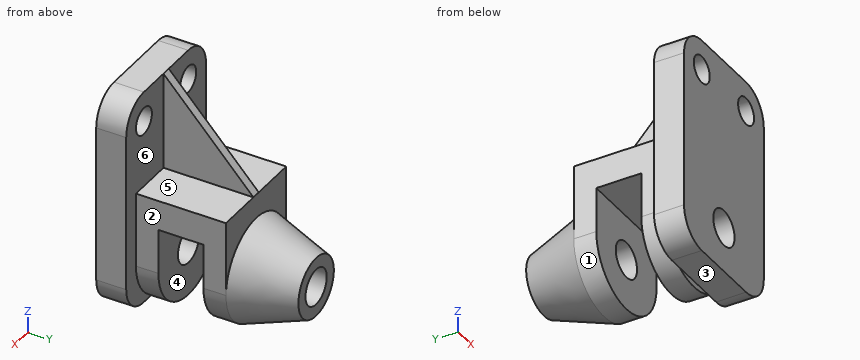
from build123d import *

# Parameters (mm, degrees)
SKETCH2_W           = 90
SKETCH2_H           = 145
SKETCH2_R           = 9
BOSS_EXTRUDE2_DEPTH = 20
FILLET1_R           = 20
FILLET2_R           = 20
BOSS_EXTRUDE3_DEPTH = 60
SKETCH4_W           = 83.251362913
SKETCH4_H           = 30
CUT_EXTRUDE1_DEPTH  = 136.98988933
SKETCH5_R           = 34
SKETCH6_R           = 20
SKETCH6_3_R         = 12
CUT_EXTRUDE2_DEPTH  = 150.255653211
RIB2_REACH          = 151.256
SKETCH9_WALL_W      = 388.970336646
SKETCH9_WALL_H      = 6


with BuildPart() as part:
    # Sketch2 → Boss-Extrude2 (new body)
    with BuildSketch(Plane(origin=(0, 0, 0), x_dir=(1, 0, 0), z_dir=(0, 1, 0))):
        Rectangle(SKETCH2_W, SKETCH2_H)
        with Locations(Location((-25, -52.5, 0), (0, 0, 270))):
            Circle(SKETCH2_R, mode=Mode.SUBTRACT)
        with Locations(Location((25, -52.5, 0), (0, 0, 270))):
            Circle(SKETCH2_R, mode=Mode.SUBTRACT)
    extrude(amount=BOSS_EXTRUDE2_DEPTH)

    # Fillet1
    fillet1_edges = [part.edges().sort_by_distance(p)[0] for p in [
        (45, 10, 72.5),
        (-45, 10, 72.5),
    ]]
    fillet(fillet1_edges, radius=FILLET1_R)

    # Fillet2
    fillet2_edges = [part.edges().sort_by_distance(p)[0] for p in [
        (-45, 10, -72.5),
        (45, 10, -72.5),
    ]]
    fillet(fillet2_edges, radius=FILLET2_R)

    # Sketch3 → Boss-Extrude3 (add)
    with BuildSketch(Plane(origin=(0, 20, 0), x_dir=(1, 0, 0), z_dir=(0, 1, 0))):
        with BuildLine():
            Line((-34, -7.5), (34, -7.5))
            Line((34, -7.5), (34, 42.5))
            ThreePointArc((34, 42.5), (0, 76.5), (-34, 42.5))
            Line((-34, 42.5), (-34, -7.5))
        make_face()
    extrude(amount=BOSS_EXTRUDE3_DEPTH)

    # Sketch4 → Cut-Extrude1 (cut, through all)
    with BuildSketch(Plane(origin=(34, 0, 0), x_dir=(0, 0, -1), z_dir=(1, 0, 0))):
        with Locations((54.125681457, 50)):
            Rectangle(SKETCH4_W, SKETCH4_H)
    extrude(amount=-CUT_EXTRUDE1_DEPTH, mode=Mode.SUBTRACT)

    # Sketch5 → Loft1 section 0
    with BuildSketch(Plane(origin=(0, 80, 0), x_dir=(1, 0, 0), z_dir=(0, 1, 0))):
        with Locations((0, 42.5)):
            Circle(SKETCH5_R)
    # Sketch6 → Loft1 section 1
    with BuildSketch(Plane(origin=(0, 120, 0), x_dir=(1, 0, 0), z_dir=(0, 1, 0))):
        with Locations((0, 42.5)):
            Circle(SKETCH6_R)
    loft()

    # Sketch6<3> → Cut-Extrude2 (cut, through all)
    with BuildSketch(Plane(origin=(0, 120, 0), x_dir=(1, 0, 0), z_dir=(0, 1, 0))):
        with Locations(Location((0, 42.5, 0), (0, 0, 270))):
            Circle(SKETCH6_3_R)
    extrude(amount=-CUT_EXTRUDE2_DEPTH, mode=Mode.SUBTRACT)

    # Sketch9 wall → Rib2 (add, up to next)
    with BuildSketch(Plane(origin=(0, 50, 40), x_dir=(0, 0.678280102733, -0.734803444627), z_dir=(0, 0.734803444627, 0.678280102733)), mode=Mode.PRIVATE) as rib2_sk1:
        Rectangle(SKETCH9_WALL_W, SKETCH9_WALL_H)
    rib2_tool1 = extrude(rib2_sk1.sketch, amount=-RIB2_REACH, mode=Mode.PRIVATE) - part.part
    add(rib2_tool1.solids().sort_by_distance((0, 50, 40))[0])


solid = part.part
Input: part model. Units: mm. Frame: model coordinates. Face numbers are marked on the shaded views. A direction names the side the tool comes from. Coordinates: 2 decimals unless noted, no trailing zeros. Order: outer loops, then holes, each group sorted by start corner. A loop starts at its lowest first (then second) coordinate and runs counter-clockwise, first axis right, second up. Notation, with made-up numbers: M 41.5,51.5 L 95.5,51.5 A15 ccw 95.5,76.5 Z; hole C -36.5,36 d7. An arc over 180 degrees is marked long. One line per question, with ' | ' between items.
Item 1: Reachability of the marked faces 1, 2 and 3 from +Z, -Z, +X, -X, +Y, -Y: full face, straight path, thin tool, end or side. Return the list, or none.
Geometry results:
face 1: -Z, +Y | face 2: +Z, -Z, +X, +Y | face 3: -Z, +X, -X, -Y
Item 2: Section A-A (x = 0). Output: boundary loops of the cut face in (y, z).
Geometry results:
outline: M 0,-72.5 L 20,-72.5 L 20,-76.5 L 35,-76.5 L 35,-54.5 L 0,-54.5 Z; M 0,-30.5 L 35,-30.5 L 35,-12.5 L 65,-12.5 L 65,-30.5 L 120,-30.5 L 120,-22.5 L 80,-8.5 L 80,7.5 L 20,72.5 L 0,72.5 Z; M 65,-76.5 L 80,-76.5 L 120,-62.5 L 120,-54.5 L 65,-54.5 Z
Item 3: Draft query along Y for the marked faces 4, 5 and 6. Return one class per face: released by +Y, released by -Y, zero draft, split by the parting line, or undercut.
Geometry results:
face 4: undercut | face 5: zero draft | face 6: released by +Y
Item 4: Section B-B (y = 15.5). Output: boundary loops of the cut face in (x, z).
Geometry results:
outline: M -45,-52.5 A20 ccw -25,-72.5 L 25,-72.5 A20 ccw 45,-52.5 L 45,52.5 A20 ccw 25,72.5 L -25,72.5 A20 ccw -45,52.5 Z; hole C -25,52.5 d18; hole C 0,-42.5 d24; hole C 25,52.5 d18
Item 5: Section C-C (y = 74). Output: boundary loops of the cut face in (x, z).
Geometry results:
outline: M -34,-42.5 A34 ccw 34,-42.5 L 34,7.5 L 3,7.5 L 3,14 L -3,14 L -3,7.5 L -34,7.5 Z; hole C 0,-42.5 d24
Item 6: Section D-D (z = 30.5). Output: boundary loops of the cut face in (x, y).
Geometry results:
outline: M -45,0 L 45,0 L 45,20 L 3,20 L 3,58.77 L -3,58.77 L -3,20 L -45,20 Z
Item 7: Pin query (flat end, axial travel): pin 1 (1 mm diameter, centred on x = 35.5, z = 35, fed in from +Y); pin 2 (3 mm diameter, centred on x = -6.5, z = -75, fed in from -Y); pin 3 (10 mm diameter, centred on x = -33.5, y = 73.5, fed in from +Z). Return the tip coordinate at first contact, or that it passes through.
Geometry results:
pin 1: stops at y = 20 | pin 2: stops at y = 20 | pin 3: stops at z = 7.5
Item 8: Ray query, line 1 along X through (y, z) = (8, 52.5); line 2 along X through (y, z) = (36, 37); line 3 along Y through (x, z) = (38.5, 30). Return the intervals inside material, ascending.
Geometry results:
line 1: x = -45 to -34, -16 to 16, 34 to 45 | line 2: x = -3 to 3 | line 3: y = 0 to 20
